Could you check a few things on this drawing? It's one solid part, dimensions in mm from its lowest x, y, z. Round coordinates to 2 decimals unless told otherwise and drop trailing zeros. Write each loop counter-clockwise with the first axis right and the second up, starting at its lowest first coordinate (ties: lowest second). Pieces come first, ordered by that corner, then holes. Notation, with made-up numbers: (53, -4.5) - (91, -4.5) arc R16 ccw to (91, 4.5) - close; hole circle Ø2 at (-30.5, 76). An arc over 180 degrees is marked (long way). Write item = value, one per line. Start each with the question number.
Item 1: If I drill on line 1 along X through (y, z) = (4.2, 10); line 2 along Z through (x, y) = (108, 4.8); line 3 along X through (y, z) = (1.7, 11.75), over which ranges is the centre line in solid material (lowest first)? Write a range as [from, to].
Item 2: If we section it at B-B (z = 10): Please give me the cut outline in (x, y), and give its area (3 significant figures).
Item 3: If we section it at C-C (y = 2): Please give me the cut outline in (x, z).
Item 4: For P1, Ø5.5, axis at x = 36, z = 10, coming from the -Y side, with a flat end and sliding along its axis, tell me the tip position at first contact or that it passes through.
Item 5: If we section it at A-A (x = 108): Please give me the cut outline in (y, z), and give its area (3 significant figures).
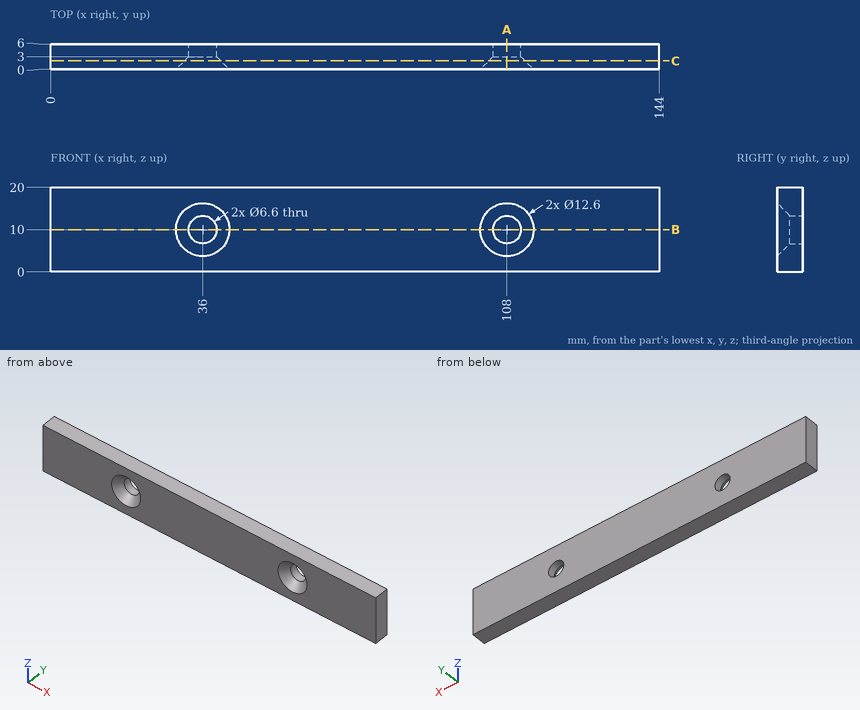
Reply:
q1.line_1 = [0, 32.7], [39.3, 104.7], [111.3, 144]
q1.line_2 = [0, 6.7], [13.3, 20]
q1.line_3 = [0, 31.75], [40.25, 103.75], [112.25, 144]
q2.outline = (0, 0) - (29.7, 0) - (32.7, 3) - (32.7, 6) - (0, 6) - close; (39.3, 3) - (42.3, 0) - (101.7, 0) - (104.7, 3) - (104.7, 6) - (39.3, 6) - close; (111.3, 3) - (114.3, 0) - (144, 0) - (144, 6) - (111.3, 6) - close
q2.area = 767 mm2
q3.outline = (0, 0) - (144, 0) - (144, 20) - (0, 20) - close; hole circle Ø8.6 at (36, 10); hole circle Ø8.6 at (108, 10)
q4.P1 = through
q5.outline = (0, 0) - (6, 0) - (6, 6.7) - (3, 6.7) - (0, 3.7) - close; (0, 16.3) - (3, 13.3) - (6, 13.3) - (6, 20) - (0, 20) - close
q5.area = 71.4 mm2
